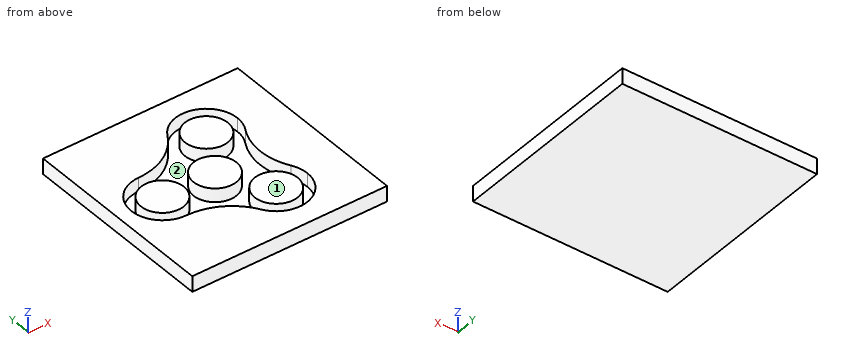
```python
from build123d import *

# Parameters (mm, degrees)
F0_W     = 100
F0_H     = 100
F1_DEPTH = 7
F0_R     = 11
F2_DEPTH = 7
F3_R     = 3.49999
F5_W     = 100
F5_H     = 100
F6_DEPTH = 1
F7_R     = 11
F8_DEPTH = 7


# Not quite as in the source:
# - a fillet or chamfer is up to 0.001 mm smaller than in the source, because OpenCascade refuses the exact size


with BuildPart() as f1:
    # F0 (on Top) → F1 (new body)
    with BuildSketch(Plane.XY):
        Rectangle(F0_W, F0_H)
        with BuildLine():
            ThreePointArc((-27, 16), (-11.6173140978, 20.1217782649), (-0.3564064606, 31.3826859022))
            ThreePointArc((-0.3564064606, 31.3826859022), (17.6411047216, 38.8374991228), (29.5, 23.3826859022))
            ThreePointArc((29.5, 23.3826859022), (28.9548132206, 19.2415811805), (27.3564064606, 15.3826859022))
            ThreePointArc((27.3564064606, 15.3826859022), (23.2346281956, 0), (27.3564064606, -15.3826859022))
            ThreePointArc((27.3564064606, -15.3826859022), (28.9548132206, -19.2415811805), (29.5, -23.3826859022))
            ThreePointArc((29.5, -23.3826859022), (17.6411047216, -38.8374991228), (-0.3564064606, -31.3826859022))
            ThreePointArc((-0.3564064606, -31.3826859022), (-11.6173140978, -20.1217782649), (-27, -16))
            ThreePointArc((-27, -16), (-43, 0), (-27, 16))
        make_face(mode=Mode.SUBTRACT)
    extrude(amount=F1_DEPTH)


with BuildPart() as f2:
    # F0 (on Top) → F2 (new body)
    with BuildSketch(Plane.XY):
        with BuildLine():
            ThreePointArc((-16, 0), (-15.3622914957, 4.472135955), (-13.5, 8.5877820187))
            ThreePointArc((-13.5, 8.5877820187), (-19.299497169, 14.0250581514), (-27, 16))
            ThreePointArc((-27, 16), (-43, 0), (-27, -16))
            ThreePointArc((-27, -16), (-19.299497169, -14.0250581514), (-13.5, -8.5877820187))
            ThreePointArc((-13.5, -8.5877820187), (-15.3622914957, -4.472135955), (-16, 0))
        make_face()
        with Locations((-27, 0)):
            Circle(F0_R, mode=Mode.SUBTRACT)
        with BuildLine():
            ThreePointArc((-0.3564064606, 31.3826859022), (-2.4963080642, 23.7263839043), (-0.6872373903, 15.9852339604))
            ThreePointArc((-0.6872373903, 15.9852339604), (3.8081625511, 15.5402026365), (8.0000002665, 13.8564063067))
            ThreePointArc((8.0000002665, 13.8564063067), (11.5541292005, 11.068066607), (14.1872373903, 7.3974519418))
            ThreePointArc((14.1872373903, 7.3974519418), (21.7958052331, 9.7013257529), (27.3564064606, 15.3826859022))
            ThreePointArc((27.3564064606, 15.3826859022), (28.9548132206, 19.2415811805), (29.5, 23.3826859022))
            ThreePointArc((29.5, 23.3826859022), (17.6411047216, 38.8374991228), (-0.3564064606, 31.3826859022))
        make_face()
        with BuildLine():
            ThreePointArc((24.5, 23.3826859022), (19.0000001332, 13.8564065375), (8.0000002665, 13.8564063067))
            ThreePointArc((8.0000002665, 13.8564063067), (7.9999998668, 32.9089652669), (24.5, 23.3826859022))
        make_face(mode=Mode.SUBTRACT)
        with BuildLine():
            ThreePointArc((-0.6872373903, 15.9852339604), (1.9458710013, 12.3146190845), (5.5000002388, 9.5262793037))
            ThreePointArc((5.5000002388, 9.5262793037), (9.6918377323, 7.8424831962), (14.1872373903, 7.3974519418))
            ThreePointArc((14.1872373903, 7.3974519418), (11.5541292005, 11.068066607), (8.0000002665, 13.8564063067))
            ThreePointArc((8.0000002665, 13.8564063067), (3.8081625511, 15.5402026365), (-0.6872373903, 15.9852339604))
        make_face()
        with BuildLine():
            ThreePointArc((27.3564064606, -15.3826859022), (21.7958052331, -9.7013257529), (14.1872373903, -7.3974519418))
            ThreePointArc((14.1872373903, -7.3974519418), (11.5541290581, -11.0680667557), (7.99999991, -13.8564065125))
            ThreePointArc((7.99999991, -13.8564065125), (3.8081623512, -15.5402026855), (-0.6872373903, -15.9852339604))
            ThreePointArc((-0.6872373903, -15.9852339604), (-2.4963080642, -23.7263839043), (-0.3564064606, -31.3826859022))
            ThreePointArc((-0.3564064606, -31.3826859022), (17.6411047216, -38.8374991228), (29.5, -23.3826859022))
            ThreePointArc((29.5, -23.3826859022), (28.9548132206, -19.2415811805), (27.3564064606, -15.3826859022))
        make_face()
        with BuildLine():
            ThreePointArc((24.5, -23.3826859022), (8.000000045, -32.9089653698), (7.99999991, -13.8564065125))
            ThreePointArc((7.99999991, -13.8564065125), (18.999999955, -13.8564064346), (24.5, -23.3826859022))
        make_face(mode=Mode.SUBTRACT)
        with BuildLine():
            ThreePointArc((14.1872373903, -7.3974519418), (9.6918376596, -7.842483214), (5.5000001093, -9.5262793785))
            ThreePointArc((5.5000001093, -9.5262793785), (1.9458709496, -12.3146191385), (-0.6872373903, -15.9852339604))
            ThreePointArc((-0.6872373903, -15.9852339604), (3.8081623512, -15.5402026855), (7.99999991, -13.8564065125))
            ThreePointArc((7.99999991, -13.8564065125), (11.5541290581, -11.0680667557), (14.1872373903, -7.3974519418))
        make_face()
        with BuildLine():
            ThreePointArc((-0.3564064606, -31.3826859022), (-2.4963080642, -23.7263839043), (-0.6872373903, -15.9852339604))
            ThreePointArc((-0.6872373903, -15.9852339604), (-8, -13.8564064606), (-13.5, -8.5877820187))
            ThreePointArc((-13.5, -8.5877820187), (-19.299497169, -14.0250581514), (-27, -16))
            ThreePointArc((-27, -16), (-11.6173140978, -20.1217782649), (-0.3564064606, -31.3826859022))
        make_face()
        with BuildLine():
            ThreePointArc((5.5000002388, 9.5262793037), (9.5262795106, 5.4999998806), (11, 0))
            ThreePointArc((11, 0), (9.5262794732, -5.4999999453), (5.5000001093, -9.5262793785))
            ThreePointArc((5.5000001093, -9.5262793785), (9.6918376596, -7.842483214), (14.1872373903, -7.3974519418))
            ThreePointArc((14.1872373903, -7.3974519418), (15.5402026731, -3.8081624017), (16, 0))
            ThreePointArc((16, 0), (15.5402026731, 3.8081624017), (14.1872373903, 7.3974519418))
            ThreePointArc((14.1872373903, 7.3974519418), (9.6918377323, 7.8424831962), (5.5000002388, 9.5262793037))
        make_face()
        with BuildLine():
            ThreePointArc((-0.6872373903, -15.9852339604), (1.9458709496, -12.3146191385), (5.5000001093, -9.5262793785))
            ThreePointArc((5.5000001093, -9.5262793785), (-5.4999999453, -9.5262794732), (-11, 0))
            ThreePointArc((-11, 0), (-11.6377085043, -4.472135955), (-13.5, -8.5877820187))
            ThreePointArc((-13.5, -8.5877820187), (-8, -13.8564064606), (-0.6872373903, -15.9852339604))
        make_face()
        with BuildLine():
            ThreePointArc((-13.5, -8.5877820187), (-11.6377085043, -4.472135955), (-11, 0))
            ThreePointArc((-11, 0), (-11.6377085043, 4.472135955), (-13.5, 8.5877820187))
            ThreePointArc((-13.5, 8.5877820187), (-15.3622914957, 4.472135955), (-16, 0))
            ThreePointArc((-16, 0), (-15.3622914957, -4.472135955), (-13.5, -8.5877820187))
        make_face()
        with BuildLine():
            ThreePointArc((-11, 0), (-5.4999998806, 9.5262795106), (5.5000002388, 9.5262793037))
            ThreePointArc((5.5000002388, 9.5262793037), (1.9458710013, 12.3146190845), (-0.6872373903, 15.9852339604))
            ThreePointArc((-0.6872373903, 15.9852339604), (-8, 13.8564064606), (-13.5, 8.5877820187))
            ThreePointArc((-13.5, 8.5877820187), (-11.6377085043, 4.472135955), (-11, 0))
        make_face()
        with BuildLine():
            ThreePointArc((-13.5, 8.5877820187), (-8, 13.8564064606), (-0.6872373903, 15.9852339604))
            ThreePointArc((-0.6872373903, 15.9852339604), (-2.4963080642, 23.7263839043), (-0.3564064606, 31.3826859022))
            ThreePointArc((-0.3564064606, 31.3826859022), (-11.6173140978, 20.1217782649), (-27, 16))
            ThreePointArc((-27, 16), (-19.299497169, 14.0250581514), (-13.5, 8.5877820187))
        make_face()
        with BuildLine():
            ThreePointArc((27.3564064606, 15.3826859022), (21.7958052331, 9.7013257529), (14.1872373903, 7.3974519418))
            ThreePointArc((14.1872373903, 7.3974519418), (15.5402026731, 3.8081624017), (16, 0))
            ThreePointArc((16, 0), (15.5402026731, -3.8081624017), (14.1872373903, -7.3974519418))
            ThreePointArc((14.1872373903, -7.3974519418), (21.7958052331, -9.7013257529), (27.3564064606, -15.3826859022))
            ThreePointArc((27.3564064606, -15.3826859022), (23.2346281956, 0), (27.3564064606, 15.3826859022))
        make_face()
    extrude(amount=F2_DEPTH)

    # F3 (radius 3.5 in the source; OpenCascade refuses exactly that, so slightly less here)
    f3_edges = [f2.edges().sort_by_distance(p)[0] for p in [
        (21.5, 37.239092, 7),
        (21.5, 37.239092, 0),
    ]]
    fillet(f3_edges, radius=F3_R)


with BuildPart() as f1_1:
    add(f1.part)

    # F4: cut F2
    add(f2.part, mode=Mode.SUBTRACT)

    # F5 (on Top) → F6 (join)
    with BuildSketch(Plane.XY):
        Rectangle(F5_W, F5_H)
    extrude(amount=-F6_DEPTH)

    # F7 (on face) → F8 (join)
    with BuildSketch(Plane.XY):
        Circle(F7_R)
        with Locations((13.5, 23.3826859022)):
            Circle(F7_R)
        with Locations((-27, 0)):
            Circle(F7_R)
        with Locations((13.5, -23.3826859022)):
            Circle(F7_R)
    extrude(amount=F8_DEPTH)


solid = f1_1.part
```
Read the model definition and answer for the solid it produces. Units are mm, in the model's axes. Face numbers are marked on the shaded views. Round coordinates to 2 decimals unless told otherwise and drop trailing zeros. Write each loop counter-clockwise with the first axis right and the second up, starting at its lowest first coordinate (ties: lowest second). Pieces come first, ordered by that corner, then holes. Notation, with made-up numbers: (47.25, 25) -> (86.25, 25) arc R18 cw to (86.25, 39) -> close; hole circle Ø8 at (82.25, 46.25). An arc over 180 degrees is marked (long way). Answer in a Markdown table with one row per item. Add a question column.
1) Find section B-B, the plane x = 13.5. Determine the outline of the cut face in (y, z).
2) Determine the mould class of the marked faces 1 and 2 for opening direction Y: pulls with the +Y half, pulls with the -Y half, needs draft (parallel to the pull), parting line crosses it, or undercut.
3) Find section D-D, the plane y = -29. Determine the outline of the cut face in (x, z), and give its area (3 significant figures).
4) Find section A-A, the plane z = 5. Determine the outline of the cut face in (x, y), and give its area (3 significant figures).
5) Find section C-C, the plane y = 0. Determine the outline of the cut face in (x, z).
6) Consider line 1 (Y direction, x = -27.5, z = 4.5); line 2 (Y direction, x = -35.5, z = 3.75); line 3 (X direction, y = 33.5, z = 4.5). Determine where each line is inside the solid, lowest interval first.
Findings below:
| question | item | result |
|---|---|---|
| 1 | outline | (-50, -1) -> (50, -1) -> (50, 7) -> (39.38, 7) -> (39.38, 0) -> (34.38, 0) -> (34.38, 7) -> (12.38, 7) -> (12.38, 0) -> (-12.38, 0) -> (-12.38, 7) -> (-34.38, 7) -> (-34.38, 0) -> (-39.38, 0) -> (-39.38, 7) -> (-50, 7) -> close |
| 2 | face 1 | needs draft |
| 2 | face 2 | undercut |
| 3 | outline | (-50, -1) -> (50, -1) -> (50, 7) -> (28.48, 7) -> (28.48, 0) -> (22.96, 0) -> (22.96, 7) -> (4.04, 7) -> (4.04, 0) -> (-1.88, 0) -> (-1.88, 7) -> (-50, 7) -> close |
| 3 | area | 720 mm² |
| 4 | outline | (-50, -50) -> (50, -50) -> (50, 50) -> (-50, 50) -> close; circle Ø22 at (-27, 0); circle Ø22 at (0, 0); circle Ø22 at (13.5, -23.38); circle Ø22 at (13.5, 23.38); hole (-27, -16) arc R30.77 cw to (-0.36, -31.38) arc R16 ccw to (27.36, -15.38) arc R30.77 cw to (27.36, 15.38) arc R16 ccw to (-0.36, 31.38) arc R30.77 cw to (-27, 16) arc R16 ccw to start |
| 4 | area | 8,010 mm² |
| 5 | outline | (-50, -1) -> (50, -1) -> (50, 7) -> (23.23, 7) -> (23.23, 0) -> (11, 0) -> (11, 7) -> (-11, 7) -> (-11, 0) -> (-16, 0) -> (-16, 7) -> (-38, 7) -> (-38, 0) -> (-43, 0) -> (-43, 7) -> (-50, 7) -> close |
| 6 | line 1 | -50 to -15.99, -10.99 to 10.99, 15.99 to 50 |
| 6 | line 2 | -50 to -13.56, -6.98 to 6.98, 13.56 to 50 |
| 6 | line 3 | -50 to 1.1, 9.18 to 17.82, 25.9 to 50 |
